```python
from build123d import *

# Parameters (mm, degrees)
BOSS_EXTRUDE1_DEPTH = 0.508
SKETCH3_R           = 0.635
CUT_EXTRUDE1_DEPTH  = 26.689183794
SKETCH5_R           = 1.143
SKETCH5_R_2         = 0.635
BOSS_EXTRUDE2_DEPTH = 0.762


with BuildPart() as part:
    # Sketch1 → Boss-Extrude1 (new body)
    with BuildSketch(Plane.XY):
        Polygon((1.27, 0), (1.27, 19.05), (3.81, 19.05), (0, 25.4), (-3.81, 19.05), (-1.27, 19.05), (-1.27, 0), align=None)
    extrude(amount=BOSS_EXTRUDE1_DEPTH)

    # Sketch3 → Cut-Extrude1 (cut, through all)
    with BuildSketch(Plane.XY.offset(0.508)):
        with Locations((0, 2.54)):
            Circle(SKETCH3_R)
    extrude(amount=-CUT_EXTRUDE1_DEPTH, mode=Mode.SUBTRACT)

    # Sketch5 → Boss-Extrude2 (add)
    with BuildSketch(Plane(origin=(0, 0, 0), x_dir=(-1, 0, 0), z_dir=(0, 0, -1))):
        with Locations(Location((0, 2.54, 0), (0, 0, 180))):
            Circle(SKETCH5_R)
        with Locations(Location((0, 2.54, 0), (0, 0, 180))):
            Circle(SKETCH5_R_2, mode=Mode.SUBTRACT)
    extrude(amount=BOSS_EXTRUDE2_DEPTH)


solid = part.part
```
Geometry: final body of the model. Coordinates: model frame, mm. Round coordinates to 2 decimals unless told otherwise and drop trailing zeros. Write each loop counter-clockwise with the first axis right and the second up, starting at its lowest first coordinate (ties: lowest second). Pieces come first, ordered by that corner, then holes.
Item 1: Section query B-B (x = -2.25). Return loops of the section in (y, z), plus the area to 3 significant figures.
Item 2: Mould query, pull axis Y, two halves, no side actions, for faces 1 (the face through (0.614, 1.576, -0.376)), 2 (the face through (-0.08, 1.91, -0.12)), 3 (the face through (0, 14, 0.508)). Classes: +Y half, -Y half, draft (parallel to the pull), parting line (faces both ways), or undercut.
Item 3: Pin query (flat end, axial travel): P1, Ø0.6, axis at y = 9, z = 0.5, coming from the +X side. Return the tip coordinate at first contact, or that it passes through.
Item 4: Section query A-A (y = 2.54). Return loops of the section in (x, z) (3 decimals), plus the area to 3 significant figures.
Item 5: Material intervals for L1, parallel to Y at x = 0, z = -0.5 (3 decimals); L2, parallel to X at y = 2.54, z = -0.4 (3 decimals); L3, parallel to X at y = 2.54, z = 0.25 (3 decimals), sorted ascending.
Item 6: Section query C-C (y = 22.5). Return loops of the section in (x, z), plus the area to 3 significant figures.
Completed:
1. outline: (19.05, 0) - (21.65, 0) - (21.65, 0.51) - (19.05, 0.51) - close
1. area: 1.32 mm2
2. face 1: parting line
2. face 2: undercut
2. face 3: draft
3. P1: stops at x = 1.27
4. outline: (-1.27, 0) - (-1.143, 0) - (-1.143, -0.762) - (-0.635, -0.762) - (-0.635, 0.508) - (-1.27, 0.508) - close; (0.635, -0.762) - (1.143, -0.762) - (1.143, 0) - (1.27, 0) - (1.27, 0.508) - (0.635, 0.508) - close
4. area: 1.42 mm2
5. L1: y = 1.397 to 1.905, 3.175 to 3.683
5. L2: x = -1.143 to -0.635, 0.635 to 1.143
5. L3: x = -1.27 to -0.635, 0.635 to 1.27
6. outline: (-1.74, 0) - (1.74, 0) - (1.74, 0.51) - (-1.74, 0.51) - close
6. area: 1.77 mm2
